```python
from build123d import *

# Parameters (mm, degrees)
SKETCH1_W           = 98.1
SKETCH1_H           = 55.8
BOSS_EXTRUDE1_DEPTH = 6
SKETCH2_W           = 5.9
SKETCH2_H           = 55.8
SKETCH2_W_2         = 6.1
CUT_EXTRUDE1_DEPTH  = 4.5
SKETCH3_W           = 14.8
SKETCH3_H           = 14.7
BOSS_EXTRUDE4_DEPTH = 4.1
SKETCH4_W           = 2.6
SKETCH4_H           = 35.7
BOSS_EXTRUDE5_DEPTH = 18.6
SKETCH5_W           = 14.8
SKETCH5_H           = 14.7
BOSS_EXTRUDE6_DEPTH = 2.2


with BuildPart() as part:
    # Sketch1 → Boss-Extrude1 (new body)
    with BuildSketch(Plane.XY):
        with Locations((0, -1.56102071)):
            Rectangle(SKETCH1_W, SKETCH1_H)
    extrude(amount=BOSS_EXTRUDE1_DEPTH)

    # Sketch2 → Cut-Extrude1 (cut)
    with BuildSketch(Plane.XY.offset(6)):
        with Locations((-46.1, -1.56102071)):
            Rectangle(SKETCH2_W, SKETCH2_H)
        with Locations((46, -1.56102071)):
            Rectangle(SKETCH2_W_2, SKETCH2_H)
    extrude(amount=-CUT_EXTRUDE1_DEPTH, mode=Mode.SUBTRACT)

    # Sketch3 → Boss-Extrude4 (add)
    with BuildSketch(Plane.XY.offset(6)):
        with Locations((-1.877850501, -21.022317242)):
            Rectangle(SKETCH3_W, SKETCH3_H)
    extrude(amount=-BOSS_EXTRUDE4_DEPTH)

    # Sketch4 → Boss-Extrude5 (add)
    with BuildSketch(Plane(origin=(0, 0, 0), x_dir=(-1, 0, 0), z_dir=(0, 0, -1))):
        with Locations((-47.75, -1.098812698)):
            Rectangle(SKETCH4_W, SKETCH4_H)
    extrude(amount=BOSS_EXTRUDE5_DEPTH)

    # Sketch5 → Boss-Extrude6 (add)
    with BuildSketch(Plane(origin=(0, 0, 0), x_dir=(-1, 0, 0), z_dir=(0, 0, -1))):
        with Locations((2.55, -20.51102071)):
            Rectangle(SKETCH5_W, SKETCH5_H)
    extrude(amount=BOSS_EXTRUDE6_DEPTH)


solid = part.part
```
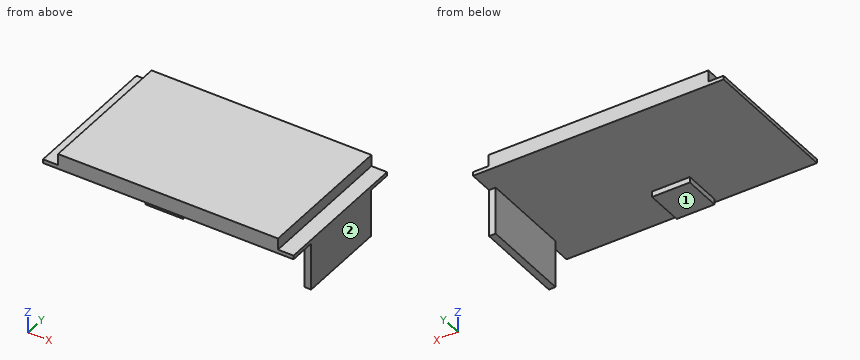
Geometry: final body of the model. Coordinates: model frame, mm. Face numbers are marked on the shaded views. A direction names the side the tool comes from. Round coordinates to 2 decimals unless told otherwise and drop trailing zeros. Loops run counter-clockwise (first coordinate to the right, second up) from the corner with the lowest first, then second, coordinate; pieces in that order, holes last. Notation, with made-up numbers: (58, 2.25) -> (63, 2.25) arc R14 ccw to (63, 12.25) -> close; hole circle Ø9 at (-8, 46). An arc over 180 degrees is marked (long way). Use one line per item in the form item = value.
Item 1: Material intervals for probe 1 along X at (y, z) = (-14, -1.5); probe 2 along Z at (x, y) = (6, -26.5); probe 3 along X at (y, z) = (7.5, -6.25), sorted ascending.
Evaluation:
probe_1 = -9.95 to 4.85, 46.45 to 49.05
probe_2 = 0 to 6
probe_3 = 46.45 to 49.05
Item 2: Cut plane B-B on z = -7.5. Output: boundary loops of the cut face in (x, y).
Evaluation:
outline = (46.45, -18.95) -> (49.05, -18.95) -> (49.05, 16.75) -> (46.45, 16.75) -> close
Item 3: Access query for the marked faces 1 and 2. Directions: +Z, -Z, +X, -X, +Y, -Y. A direction counts if a zero-diameter tool reaches every point of the face in a straight line with its end or side. Return the directions, or none.
Evaluation:
face_1 = -Z, -X, +Y, -Y
face_2 = +Z, -Z, +X, +Y, -Y
Item 4: Cut plane A-A on y = 13. Output: boundary loops of the cut face in (x, z).
Evaluation:
outline = (-49.05, 0) -> (46.45, 0) -> (46.45, -18.6) -> (49.05, -18.6) -> (49.05, 1.5) -> (42.95, 1.5) -> (42.95, 6) -> (-43.15, 6) -> (-43.15, 1.5) -> (-49.05, 1.5) -> close
Item 5: Contact query for flat-ended pins moving along their axis: pin 1 Ø4 at (x, y) = (-1.5, 19) entering from -Z; pin 2 Ø1.3 at (y, z) = (5, 4.5) entering from +X; pin 3 Ø1.8 at (x, y) = (47, -3) entering from +Z; pin 4 Ø2 at (x, z) = (-6.5, -4) entering from -Y. Output: stop coordinate, or through.
Evaluation:
pin_1 = 0
pin_2 = 42.95
pin_3 = 1.5
pin_4 = through
Item 6: Cut plane C-C on x = 17.5. Output: boundary loops of the cut face in (y, z).
Evaluation:
outline = (-29.46, 0) -> (26.34, 0) -> (26.34, 6) -> (-29.46, 6) -> close
